from build123d import *

# Parameters (mm, degrees)
F0_W     = 8.128
F0_H     = 63.5
F0_W_2   = 63.5
F0_H_2   = 8.128
F1_DEPTH = 3
F2_R     = 5.08


with BuildPart() as f1:
    # F0 (on Top) → F1 (new body)
    with BuildSketch(Plane.XY):
        Polygon((77.085001, 76.752045), (-72.914999, 76.752045), (-72.914999, -73.247955), align=None)
        with Locations((-53.864999, 6.902045)):
            Rectangle(F0_W, F0_H, mode=Mode.SUBTRACT)
        with Locations((-3.064999, 57.702045)):
            Rectangle(F0_W_2, F0_H_2, mode=Mode.SUBTRACT)
    extrude(amount=F1_DEPTH)

    # F2
    f2_edges = [f1.edges().sort_by_distance(p)[0] for p in [
        (-72.914999, -73.247955, 1.5),
        (77.085001, 76.752045, 1.5),
    ]]
    fillet(f2_edges, radius=F2_R)


solid = f1.part
Work out the finished part from the listing and answer in its coordinate system (mm). Round coordinates to 2 decimals unless told otherwise and drop trailing zeros. Write each loop counter-clockwise with the first axis right and the second up, starting at its lowest first coordinate (ties: lowest second). Pieces come first, ordered by that corner, then holes. Notation, with made-up numbers: M -26,29 L 32,29 A13 cw 32,53 Z; hole C 6,56 d10. An arc over 180 degrees is marked long. Use a Markdown table: item, result.
1) Consider line 1 (X direction, y = 38.5, z = 1.9) (3 decimals); line 2 (X direction, y = -14, z = 0.35) (3 decimals); line 3 (Y direction, x = 14.5, z = 2.4). Determine where each line is inside the solid, lowest interval first. Write a range as [from, to].
Taken from the geometry:
| item | result |
|---|---|
| line 1 | x = [-72.915, -57.929], [-49.801, 38.833] |
| line 2 | x = [-72.915, -57.929], [-49.801, -13.667] |
| line 3 | y = [14.17, 53.64], [61.77, 76.75] |
2) Flat-ended cylindrical pins translate along their axes: pin 1 (1.5 mm diameter, centred on y = 59.5, z = 2, fed in from +X); pin 2 (1.5 mm diameter, centred on x = -54, z = 2, fed in from -Y); pin 3 (0.9 mm diameter, centred on x = -13, z = 1.5, fed in from -Y). Find the tip coordinate at first contact, or state that the pin passes through.
Taken from the geometry:
| item | result |
|---|---|
| pin 1 | stops at x = 60.58 |
| pin 2 | stops at y = -55.08 |
| pin 3 | stops at y = -13.78 |
3) The part is cut by section A-A on z = 1.2. Give the vertices of the cut face in (x, y) (3 decimals).
Taken from the geometry:
| item | result |
|---|---|
| outline | M -72.915,-60.984 A5.08 ccw -64.243,-64.576 L 68.413,68.08 A5.08 ccw 64.821,76.752 L -72.915,76.752 Z; hole M -57.929,-24.848 L -49.801,-24.848 L -49.801,38.652 L -57.929,38.652 Z; hole M -34.815,53.638 L 28.685,53.638 L 28.685,61.766 L -34.815,61.766 Z |
4) The part is cut by section D-D on x = 55.5. Give the vertices of the cut face in (y, z), plus the area to 3 significant figures.
Taken from the geometry:
| item | result |
|---|---|
| outline | M 55.17,0 L 76.75,0 L 76.75,3 L 55.17,3 Z |
| area | 64.8 mm2 |
5) The part is cut by section B-B on x = 1. Give the vertices of the cut face in (y, z).
Taken from the geometry:
| item | result |
|---|---|
| outline | M 0.67,0 L 53.64,0 L 53.64,3 L 0.67,3 Z; M 61.77,0 L 76.75,0 L 76.75,3 L 61.77,3 Z |
6) The part is cut by section C-C on y = 15.5. Give the vertices of the cut face in (x, z) (3 decimals), plus the area to 3 significant figures.
Taken from the geometry:
| item | result |
|---|---|
| outline | M -72.915,0 L -57.929,0 L -57.929,3 L -72.915,3 Z; M -49.801,0 L 15.833,0 L 15.833,3 L -49.801,3 Z |
| area | 242 mm2 |
